from build123d import *

# Parameters (mm, degrees)
EXTRUDE_1_DEPTH = 3
EXTRUDE_2_DEPTH = 15


with BuildPart() as part:
    # 草图1 → 凸台-拉伸1 (new body)
    with BuildSketch(Plane(origin=(0, 0, 0), x_dir=(1, 0, 0), z_dir=(0, 1, 0))):
        Polygon((3, 40), (0, 40), (3, 37), align=None)
        Polygon((0, 40), (40, 0), (0, 0), align=None)
        Polygon((37, 3), (40, 0), (40, 3), align=None)
    extrude(amount=EXTRUDE_1_DEPTH)

    # 草图2 → 凸台-拉伸2 (add)
    with BuildSketch(Plane(origin=(0, 3, 0), x_dir=(1, 0, 0), z_dir=(0, 1, 0))):
        Polygon((3, 3), (3, 40), (0, 40), (0, 0), (40, 0), (40, 3), align=None)
    extrude(amount=EXTRUDE_2_DEPTH)


solid = part.part
Source: CAD feature listing. Evaluate the final solid. Frame: model axes, mm. A direction names the side the tool comes from. Coordinates: 2 decimals unless noted, no trailing zeros. Loops run counter-clockwise (first coordinate to the right, second up) from the corner with the lowest first, then second, coordinate; pieces in that order, holes last. Notation, with made-up numbers: (11.5, 22) - (17.5, 22) arc R10 cw to (17.5, 34) - close; hole circle Ø5 at (84, 44.5). An arc over 180 degrees is marked (long way). One line per question, with ' | ' between items.
1) Section D-D, the plane x = 37.5. Return loops of the section in (y, z).
Report:
outline: (0, -3) - (18, -3) - (18, 0) - (0, 0) - close
2) Section B-B, the plane y = 2. Return loops of the section in (x, z), then the cut area to 3 significant figures.
Report:
outline: (0, -40) - (3, -40) - (3, -37) - (37, -3) - (40, -3) - (40, 0) - (0, 0) - close | area: 809 mm²
3) First-contact query: P1, Ø9, axis at y = 10, z = -16.5, coming from the +X side; P2, Ø1, axis at y = 14, z = -29, coming from the -X side; P3, Ø6, axis at x = 11, z = -25, coming from the +Y side; P4, Ø5.5, axis at x = 19, y = 6.5, coming from the -Z side. Flat tips, straight axial feed; report the tip coordinate or a pass-through.
Report:
P1: stops at x = 3 | P2: stops at x = 0 | P3: stops at y = 3 | P4: stops at z = -3
4) Line query: line 1 along Z through (x, y) = (9.5, 13.5); line 2 along X through (y, z) = (16.25, -26). Output: solid intervals per line, ascending.
Report:
line 1: z = -3 to 0 | line 2: x = 0 to 3
5) Section A-A, the plane x = 30.5. Return loops of the section in (y, z), then the cut area to 3 significant figures.
Report:
outline: (0, -9.5) - (3, -9.5) - (3, -3) - (18, -3) - (18, 0) - (0, 0) - close | area: 73.5 mm²
6) Section C-C, the plane z = -14. Return loops of the section in (x, y), then the cut area to 3 significant figures.
Report:
outline: (0, 0) - (26, 0) - (26, 3) - (3, 3) - (3, 18) - (0, 18) - close | area: 123 mm²
7) Pull-direction query (X, two-part tool) for faces 1 (the face through (11, 0, -11)), 2 (the face through (3, 11, -21)), 3 (the face through (0, 9, -20)); classes: released by +X, released by -X, zero draft, split by the parting line, or undercut.
Report:
face 1: zero draft | face 2: released by +X | face 3: released by -X
8) Set-up query: faces 4 (the face through (22, 11, -3)), 5 (the face through (2, 9, -40)). Return all of +Z, -Z, +X, -X, +Y, -Y with unobstructed straight access to the full face (end or side cutting, diameter ignored); none if empty.
Report:
face 4: -Z, +X, +Y | face 5: -Z, +X, -X, +Y, -Y
